```python
from build123d import *

# Parameters (mm, degrees)
BOX_FOOTPRINT_200_X_50_MM_W                      = 200
BOX_FOOTPRINT_200_X_50_MM_H                      = 50
BOX_HEIGHT_50_MM_DEPTH                           = 50
REAR_OPENING_194_X_44_MM_W                       = 194
REAR_OPENING_194_X_44_MM_H                       = 44
REAR_CAVITY_WALL_3_MM_DEPTH                      = 47
CHASSIS_FACE_OPENINGS_AND_MOUNTING_CROSS_W       = 37
CHASSIS_FACE_OPENINGS_AND_MOUNTING_CROSS_H       = 44
CHASSIS_FACE_OPENINGS_AND_MOUNTING_CROSS_W_2     = 100
CHASSIS_FACE_OPENINGS_AND_MOUNTING_CROSS_H_2     = 13
OPEN_FRONT_MOUNTING_FRAME_DEPTH                  = 3
PHOTO_RAILS_10_X_10_PITCH_110_PROVISIONA_W       = 10
PHOTO_RAILS_10_X_10_PITCH_110_PROVISIONA_H       = 10
TWO_FORWARD_RAILS_65_MM_PROVISIONAL_DEPTH        = 65
LEFT_INWARD_PCB_MOUNTING_EAR_W                   = 10
LEFT_INWARD_PCB_MOUNTING_EAR_H                   = 10
LEFT_PCB_EAR_12_5_MM_DEPTH                       = 12.5
RIGHT_INWARD_PCB_MOUNTING_EAR_W                  = 10
RIGHT_INWARD_PCB_MOUNTING_EAR_H                  = 10
RIGHT_PCB_EAR_12_5_MM_DEPTH                      = 12.5
OPEN_FRAME_TRANSVERSE_BRACE_8_X_3_MM_W           = 3
OPEN_FRAME_TRANSVERSE_BRACE_8_X_3_MM_H           = 8
TRANSVERSE_FRAME_BRACE_DEPTH                     = 100
F_4X_VERTICAL_SLOTS_3_4_X_10_MM_DEPTH            = 3
PCB_REAR_HOLES_PITCH_85_MM_R                     = 1.7
PCB_ROOF_HOLES_DIAMETER_3_4_MM_DEPTH             = 3
PCB_FRONT_HOLES_ROW_SPACING_60_MM_R              = 1.7
PCB_EAR_HOLES_DIAMETER_3_4_MM_DEPTH              = 10
CHASSIS_TOP_HOLES_110_X_40_PROVISIONAL_R         = 1.7
F_4X_RAIL_HOLES_THROUGH_UPPER_AND_LOWER_FA_DEPTH = 10


with BuildPart() as part:
    # Box footprint 200 x 50 mm → Box height 50 mm (new body)
    with BuildSketch(Plane.XY):
        with Locations((0, 25)):
            Rectangle(BOX_FOOTPRINT_200_X_50_MM_W, BOX_FOOTPRINT_200_X_50_MM_H)
    extrude(amount=BOX_HEIGHT_50_MM_DEPTH)

    # Rear opening 194 x 44 mm → Rear cavity wall 3 mm (cut)
    with BuildSketch(Plane(origin=(0, 50, 0), x_dir=(1, 0, 0), z_dir=(0, 1, 0))):
        with Locations((0, -25)):
            Rectangle(REAR_OPENING_194_X_44_MM_W, REAR_OPENING_194_X_44_MM_H)
    extrude(amount=-REAR_CAVITY_WALL_3_MM_DEPTH, mode=Mode.SUBTRACT)

    # Chassis face openings and mounting crossbar → Open front mounting frame (cut)
    with BuildSketch(Plane.XZ):
        with Locations((-78.5, 25)):
            Rectangle(CHASSIS_FACE_OPENINGS_AND_MOUNTING_CROSS_W, CHASSIS_FACE_OPENINGS_AND_MOUNTING_CROSS_H)
        with Locations((78.5, 25)):
            Rectangle(CHASSIS_FACE_OPENINGS_AND_MOUNTING_CROSS_W, CHASSIS_FACE_OPENINGS_AND_MOUNTING_CROSS_H)
        with Locations((0, 9.5)):
            Rectangle(CHASSIS_FACE_OPENINGS_AND_MOUNTING_CROSS_W_2, CHASSIS_FACE_OPENINGS_AND_MOUNTING_CROSS_H_2)
        with Locations((0, 40.5)):
            Rectangle(CHASSIS_FACE_OPENINGS_AND_MOUNTING_CROSS_W_2, CHASSIS_FACE_OPENINGS_AND_MOUNTING_CROSS_H_2)
    extrude(amount=-OPEN_FRONT_MOUNTING_FRAME_DEPTH, mode=Mode.SUBTRACT)

    # Photo rails 10 x 10 pitch 110 provisional → Two forward rails 65 mm provisional (add)
    with BuildSketch(Plane.XZ):
        with Locations((-55, 45)):
            Rectangle(PHOTO_RAILS_10_X_10_PITCH_110_PROVISIONA_W, PHOTO_RAILS_10_X_10_PITCH_110_PROVISIONA_H)
        with Locations((55, 45)):
            Rectangle(PHOTO_RAILS_10_X_10_PITCH_110_PROVISIONA_W, PHOTO_RAILS_10_X_10_PITCH_110_PROVISIONA_H)
    extrude(amount=TWO_FORWARD_RAILS_65_MM_PROVISIONAL_DEPTH)

    # Left inward PCB mounting ear → Left PCB ear 12.5 mm (add)
    with BuildSketch(Plane(origin=(-50, 0, 0), x_dir=(0, 0, -1), z_dir=(1, 0, 0))):
        with Locations((-45, -20)):
            Rectangle(LEFT_INWARD_PCB_MOUNTING_EAR_W, LEFT_INWARD_PCB_MOUNTING_EAR_H)
    extrude(amount=LEFT_PCB_EAR_12_5_MM_DEPTH)

    # Right inward PCB mounting ear → Right PCB ear 12.5 mm (add)
    with BuildSketch(Plane.ZY.offset(-50)):
        with Locations((45, -20)):
            Rectangle(RIGHT_INWARD_PCB_MOUNTING_EAR_W, RIGHT_INWARD_PCB_MOUNTING_EAR_H)
    extrude(amount=RIGHT_PCB_EAR_12_5_MM_DEPTH)

    # Open frame transverse brace 8 x 3 mm → Transverse frame brace (add)
    with BuildSketch(Plane(origin=(-50, 0, 0), x_dir=(0, 0, -1), z_dir=(1, 0, 0))):
        with Locations((-48.5, -31)):
            Rectangle(OPEN_FRAME_TRANSVERSE_BRACE_8_X_3_MM_W, OPEN_FRAME_TRANSVERSE_BRACE_8_X_3_MM_H)
    extrude(amount=TRANSVERSE_FRAME_BRACE_DEPTH)

    # Chassis slot centers -50 -20 20 50 mm → 4x vertical slots 3.4 x 10 mm (cut)
    with BuildSketch(Plane.XZ):
        with BuildLine():
            Line((-51.7, 21.7), (-51.7, 28.3))
            ThreePointArc((-51.7, 28.3), (-50, 30), (-48.3, 28.3))
            Line((-48.3, 28.3), (-48.3, 21.7))
            ThreePointArc((-48.3, 21.7), (-50, 20), (-51.7, 21.7))
        make_face()
        with BuildLine():
            Line((-21.7, 21.7), (-21.7, 28.3))
            ThreePointArc((-21.7, 28.3), (-20, 30), (-18.3, 28.3))
            Line((-18.3, 28.3), (-18.3, 21.7))
            ThreePointArc((-18.3, 21.7), (-20, 20), (-21.7, 21.7))
        make_face()
        with BuildLine():
            Line((18.3, 21.7), (18.3, 28.3))
            ThreePointArc((18.3, 28.3), (20, 30), (21.7, 28.3))
            Line((21.7, 28.3), (21.7, 21.7))
            ThreePointArc((21.7, 21.7), (20, 20), (18.3, 21.7))
        make_face()
        with BuildLine():
            Line((48.3, 21.7), (48.3, 28.3))
            ThreePointArc((48.3, 28.3), (50, 30), (51.7, 28.3))
            Line((51.7, 28.3), (51.7, 21.7))
            ThreePointArc((51.7, 21.7), (50, 20), (48.3, 21.7))
        make_face()
    extrude(amount=-F_4X_VERTICAL_SLOTS_3_4_X_10_MM_DEPTH, mode=Mode.SUBTRACT)

    # PCB rear holes pitch 85 mm → PCB roof holes diameter 3.4 mm (cut)
    with BuildSketch(Plane.XY.offset(50)):
        with Locations((-42.5, 40)):
            Circle(PCB_REAR_HOLES_PITCH_85_MM_R)
        with Locations((42.5, 40)):
            Circle(PCB_REAR_HOLES_PITCH_85_MM_R)
    extrude(amount=-PCB_ROOF_HOLES_DIAMETER_3_4_MM_DEPTH, mode=Mode.SUBTRACT)

    # PCB front holes row spacing 60 mm → PCB ear holes diameter 3.4 mm (cut)
    with BuildSketch(Plane.XY.offset(50)):
        with Locations((-42.5, -20)):
            Circle(PCB_FRONT_HOLES_ROW_SPACING_60_MM_R)
        with Locations((42.5, -20)):
            Circle(PCB_FRONT_HOLES_ROW_SPACING_60_MM_R)
    extrude(amount=-PCB_EAR_HOLES_DIAMETER_3_4_MM_DEPTH, mode=Mode.SUBTRACT)

    # Chassis top holes 110 x 40 provisional → 4x rail holes through upper and lower faces (cut)
    with BuildSketch(Plane.XY.offset(50)):
        with Locations((-55, -55)):
            Circle(CHASSIS_TOP_HOLES_110_X_40_PROVISIONAL_R)
        with Locations((-55, -15)):
            Circle(CHASSIS_TOP_HOLES_110_X_40_PROVISIONAL_R)
        with Locations((55, -55)):
            Circle(CHASSIS_TOP_HOLES_110_X_40_PROVISIONAL_R)
        with Locations((55, -15)):
            Circle(CHASSIS_TOP_HOLES_110_X_40_PROVISIONAL_R)
    extrude(amount=-F_4X_RAIL_HOLES_THROUGH_UPPER_AND_LOWER_FA_DEPTH, mode=Mode.SUBTRACT)


solid = part.part
```
CAD build for the part. Positions are in the model's coordinates, mm. A direction names the side the tool comes from. Round coordinates to 2 decimals unless told otherwise and drop trailing zeros. Order: outer loops, then holes, each group sorted by start corner. A loop starts at its lowest first (then second) coordinate and runs counter-clockwise, first axis right, second up. Notation, with made-up numbers: (13, 83) - (63, 83) arc R20 cw to (63, 94) - close; hole circle Ø8 at (72.5, -36.5). An arc over 180 degrees is marked (long way). Answer in a Markdown table with one row per item. Add a question column.
(1) Band-saw the part on B-B on z = 6.5. List the corners of the cut face in (x, y).
(2) Drop flat-ended pins along their axis: pin 1 Ø3 at (y, z) = (-51, 42.5) entering from -X; pin 2 Ø18 at (x, y) = (54, -19.5) entering from -Z; pin 3 Ø10 at (x, z) = (-62.5, 44) entering from +Y. Give the stop position or say it passes through.
(3) 3-axis set-ups, long thin cutter, end or side, ignore diameter. For faces 4 (the face through (-1, 3, 25)), 5 (the face through (-44, -15, 45)), 6 (the face through (-50, -6, 44)): which of +Z, -Z, +X, -X, +Y, -Y reach the whole face in a straight line?
(4) Mould opens along Z. For faces 1 (the face through (-50, -45, 45)), 2 (the face through (-1, 19, 50)), 3 (the face through (-1, 25, 3)) say: +Z half, -Z half, draft (parallel to the pull), parting line (faces both ways), or undercut.
(5) Band-saw the part on C-C on x = -1. List the corners of the cut face in (y, z).
(6) Probe L1, parallel to Y at x = 55, z = 46; L2, parallel to Z at x = 27.5, y = 41; L3, parallel to X at y = 12, z = 21. List the from-to ranges inside material, lowest first. Write a range as [from, to].
(7) Band-saw the part on A-A on x = -73.5. List the corners of the cut face in (y, z).
Data:
| question | item | result |
|---|---|---|
| 1 | outline | (-100, 0) - (-97, 0) - (-97, 50) - (-100, 50) - close; (-60, 0) - (-50, 0) - (-50, 3) - (-60, 3) - close; (50, 0) - (60, 0) - (60, 3) - (50, 3) - close; (97, 0) - (100, 0) - (100, 50) - (97, 50) - close |
| 2 | pin 1 | stops at x = -60 |
| 2 | pin 2 | stops at z = 40 |
| 2 | pin 3 | stops at y = 50 |
| 3 | face 4 | +Y |
| 3 | face 5 | +Z, -Z |
| 3 | face 6 | none |
| 4 | face 1 | draft |
| 4 | face 2 | +Z half |
| 4 | face 3 | undercut |
| 5 | outline | (-35, 47) - (-27, 47) - (-27, 50) - (-35, 50) - close; (0, 0) - (50, 0) - (50, 3) - (0, 3) - close; (0, 16) - (3, 16) - (3, 34) - (0, 34) - close; (0, 47) - (50, 47) - (50, 50) - (0, 50) - close |
| 6 | L1 | y = [-65, -56.7], [-53.3, -16.7], [-13.3, 3] |
| 6 | L2 | z = [0, 3], [47, 50] |
| 6 | L3 | x = [-100, -97], [97, 100] |
| 7 | outline | (0, 0) - (50, 0) - (50, 3) - (0, 3) - close; (0, 47) - (50, 47) - (50, 50) - (0, 50) - close |
